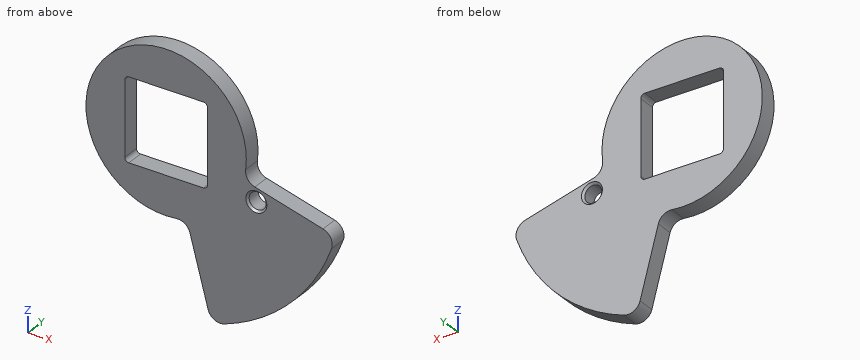
```python
from build123d import *

# Parameters (mm, degrees)
SKETCH3_R           = 2.159
BOSS_EXTRUDE1_DEPTH = 4.445
CHAMFER1_SIZE       = 0.508


with BuildPart() as part:
    # Sketch3 → Boss-Extrude1 (new body)
    with BuildSketch(Plane(origin=(0, 0, 0), x_dir=(1, 0, 0), z_dir=(0, 1, 0))):
        with BuildLine():
            Line((10.651103406, 39.750459069), (6.025173957, 22.486255331))
            ThreePointArc((6.025173957, 22.486255331), (4.728428182, 20.672198197), (2.558581153, 20.158275285))
            ThreePointArc((2.558581153, 20.158275285), (-14.368409794, -14.368409794), (20.158275285, 2.558581153))
            ThreePointArc((20.158275285, 2.558581153), (20.672198197, 4.728428182), (22.486255331, 6.025173957))
            Line((22.486255331, 6.025173957), (39.750459069, 10.651103406))
            ThreePointArc((39.750459069, 10.651103406), (41.737404706, 12.237427719), (41.923224647, 14.773142359))
            ThreePointArc((41.923224647, 14.773142359), (31.430896424, 31.430896424), (14.773142359, 41.923224647))
            ThreePointArc((14.773142359, 41.923224647), (12.237427719, 41.737404706), (10.651103406, 39.750459069))
        make_face()
        with Locations((22.86, 9.525)):
            Circle(SKETCH3_R, mode=Mode.SUBTRACT)
        with BuildLine():
            Line((-9.4615, -10.4775), (9.4615, -10.4775))
            ThreePointArc((9.4615, -10.4775), (10.17992049, -10.17992049), (10.4775, -9.4615))
            Line((10.4775, -9.4615), (10.4775, 9.4615))
            ThreePointArc((10.4775, 9.4615), (10.17992049, 10.17992049), (9.4615, 10.4775))
            Line((9.4615, 10.4775), (-9.4615, 10.4775))
            ThreePointArc((-9.4615, 10.4775), (-10.17992049, 10.17992049), (-10.4775, 9.4615))
            Line((-10.4775, 9.4615), (-10.4775, -9.4615))
            ThreePointArc((-10.4775, -9.4615), (-10.17992049, -10.17992049), (-9.4615, -10.4775))
        make_face(mode=Mode.SUBTRACT)
    extrude(amount=BOSS_EXTRUDE1_DEPTH)

    # Chamfer1
    chamfer1_edges = [part.edges().sort_by_distance(p)[0] for p in [
        (20.701, 0, -9.525),
        (20.701, 4.445, -9.525),
    ]]
    chamfer(chamfer1_edges, length=CHAMFER1_SIZE)


solid = part.part
```
The model under review builds one solid part; all positions refer to its coordinate system, in mm. Round coordinates to 2 decimals unless told otherwise and drop trailing zeros. Loops run counter-clockwise (first coordinate to the right, second up) from the corner with the lowest first, then second, coordinate; pieces in that order, holes last.
Item 1: Take a section at C-C (y = 2.8). Give the number of separate pieces and of enclosed holes in the cut face, then the cut area to 3 significant figures.
Determined:
separate pieces: 1
enclosed holes: 2
area: 1,660 mm2
Item 2: For line 1 (Z direction, x = 22.86, y = 1.7); line 2 (X direction, y = 3.5, z = 2.5); line 3 (Z direction, x = 23.5, y = 3.7), list the stretches that pass through material, from the lowest coordinate up.
Determined:
line 1: z = -38.12 to -11.68, -7.37 to -6.13
line 2: x = -20.17 to -10.48, 10.48 to 20.17
line 3: z = -37.73 to -11.59, -7.46 to -6.3
Item 3: Take a section at B-B (x = 0). Write out the cut boundary in (y, z) (1 decimal).
Determined:
outline: (0, -20.3) - (4.4, -20.3) - (4.4, -10.5) - (0, -10.5) - close; (0, 10.5) - (4.4, 10.5) - (4.4, 20.3) - (0, 20.3) - close
Item 4: Take a section at A-A (z = 0). Write out the cut boundary in (x, y) (1 decimal).
Determined:
outline: (-20.3, 0) - (-10.5, 0) - (-10.5, 4.4) - (-20.3, 4.4) - close; (10.5, 0) - (20.3, 0) - (20.3, 4.4) - (10.5, 4.4) - close
Item 5: Take a section at D-D (x = 31). Write out the cut boundary in (y, z) (3 decimals).
Determined:
outline: (0, -31.856) - (4.445, -31.856) - (4.445, -8.306) - (0, -8.306) - close
